Can you work these out from the drawing? Everything is in mm from the part's minimum corner. Round coordinates to 2 decimals unless told otherwise and drop trailing zeros. Order: outer loops, then holes, each group sorted by start corner. A loop starts at its lowest first (then second) coordinate and runs counter-clockwise, first axis right, second up. Notation, with made-up numbers: (59.25, 35) - (74.25, 35) arc R23 ccw to (74.25, 57) - close; hole circle Ø3 at (-16.75, 42.25). An arc over 180 degrees is marked (long way). Write item = value, one per line.
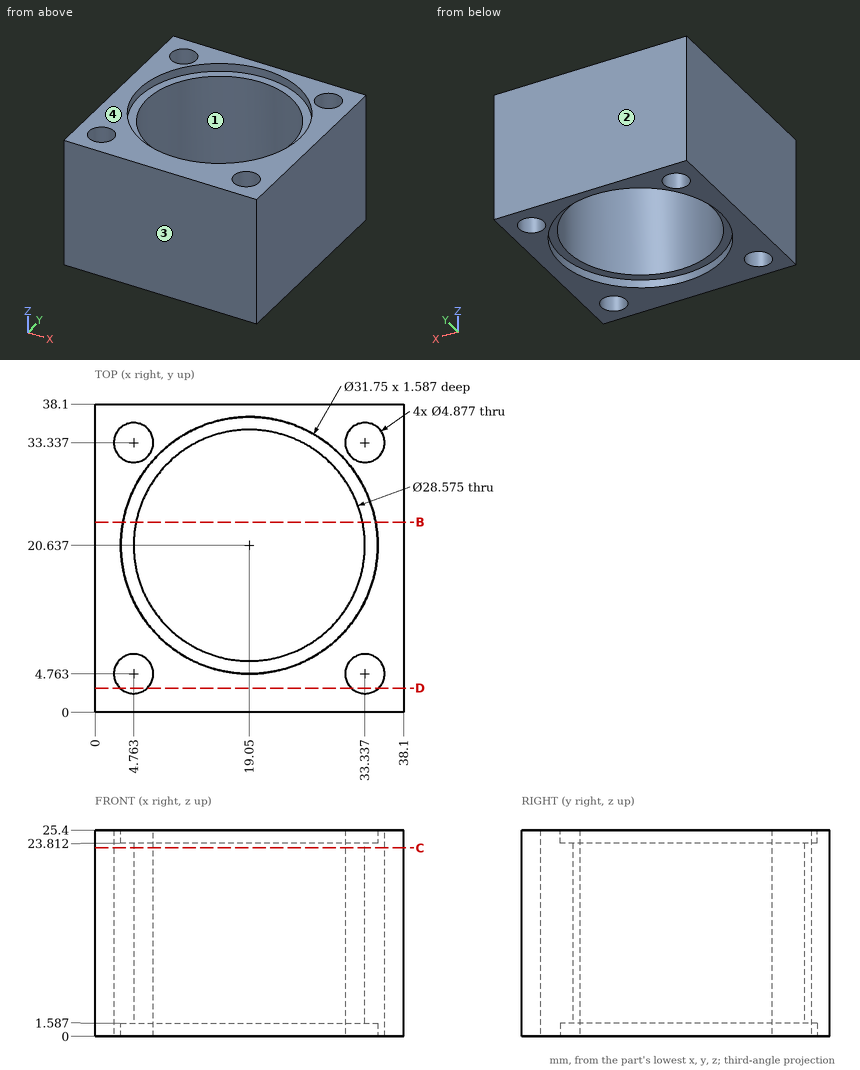
(1) Will this pin go through, and if not, where does the flat tip stop? P1, Ø8, axis at x = 28.5, y = 27, coming from the +Z side.
Computed:
P1 = 23.81
(2) If we section it at B-B (y = 23.5): Write out the boundary of the cut face in (x, z) (1 decimal).
Computed:
outline = (0, 0) - (3.4, 0) - (3.4, 1.6) - (5.1, 1.6) - (5.1, 23.8) - (3.4, 23.8) - (3.4, 25.4) - (0, 25.4) - close; (33, 1.6) - (34.7, 1.6) - (34.7, 0) - (38.1, 0) - (38.1, 25.4) - (34.7, 25.4) - (34.7, 23.8) - (33, 23.8) - close
(3) Thinking about a two-plate mould opening in Y: for the marked faces 1, 2, 3 and 4, which applies, +Y half, -Y half, draft (parallel to the pull), parting line (faces both ways), or undercut?
Computed:
face_1 = undercut
face_2 = +Y half
face_3 = -Y half
face_4 = draft
(4) If we section it at D-D (y = 3): Write out the boundary of the cut face in (x, z).
Computed:
outline = (0, 0) - (3.08, 0) - (3.08, 25.4) - (0, 25.4) - close; (6.45, 0) - (31.65, 0) - (31.65, 25.4) - (6.45, 25.4) - close; (35.02, 0) - (38.1, 0) - (38.1, 25.4) - (35.02, 25.4) - close
(5) If we section it at C-C (z = 23.25): State how many separate pieces and enclosed holes the cut face has.
Computed:
separate_pieces = 1
enclosed_holes = 5
(6) If I drill on line 1 (X direction, y = 35, z = 12) (1 decimal); line 2 (Y direction, x = 19.05, z = 0.85); line 3 (X direction, y = 20.5, z = 21.5), over which ranges is the centre line in solid material (lowest first)? Write a range as from..to.
Computed:
line_1 = 0..3, 6.5..31.6, 35.1..38.1
line_2 = 0..4.76, 36.51..38.1
line_3 = 0..4.76, 33.34..38.1
